Autodesk Inventor part; units mm, degrees
ref_plane "YZ Plane" through (0, 0, 0) normal (1, 0, 0) x (0, 1, 0)
ref_plane "XZ Plane" through (0, 0, 0) normal (0, 1, 0) x (-1, 0, 0)
ref_plane "XY Plane" through (0, 0, 0) normal (0, 0, 1) x (1, 0, 0)
sketch "Эскиз1" plane through (0, 0, 0) normal (0, 0, 1) x (1, 0, 0)
  line L0 (-25, 0) -> (25, 0) construction
  line L1 (-10, -2) -> (10, -2)
  line L2 (10, -2) -> (10, 2)
  line L3 (10, 2) -> (-10, 2)
  line L4 (-10, 2) -> (-10, -2)
  line L5 (-24, 5) -> (-20, 5)
  line L6 (-20, 5) -> (-20, -5)
  line L7 (-20, -5) -> (-24, -5)
  line L8 (-24, -5) -> (-24, 5)
  line L9 (0, 20) -> (0, -20) construction
  line L10 (24, 5) -> (20, 5)
  line L11 (20, 5) -> (20, -5)
  line L12 (20, -5) -> (24, -5)
  line L13 (24, -5) -> (24, 5)
  line L14 (-21, 20) -> (21, 20)
  line L15 (21, 20) -> (21, -20) construction
  line L16 (21, -20) -> (-21, -20)
  line L17 (-21, -20) -> (-21, 20) construction
  arc A0 (-21, 20) -> (-26, 15) centre (-21, 15) ccw
  arc A1 (-26, -15) -> (-21, -20) centre (-21, -15) ccw
  arc A2 (21, -20) -> (26, -15) centre (21, -15) ccw
  arc A3 (26, 15) -> (21, 20) centre (21, 15) ccw
  line L18 (-26, 15) -> (-26, -15)
  line L19 (26, -15) -> (26, 15)
  point P0 (0, 0)
  point P1 (-20, 0)
  point P2 (-10, 0)
  point P3 (0, -2)
  point P4 (0, 0)
  dimension "d0" = 4
  dimension "d1" = 40
  dimension "d2" = 20
  dimension "d3" = 10
  dimension "d4" = 50
  dimension "d6" = 52
  dimension "d7" = 40
  dimension "d8" = 5
extrude "Выдавливание1" add sketch "Эскиз1" along normal blind 4
properties part number "PistonPart5" material "Дерево (вишня)"
Here's how the part is built. I have some questions about the finished solid (model axes, mm). A direction names the side the tool comes from. Coordinates: 2 decimals unless noted, no trailing zeros. Write each loop counter-clockwise with the first axis right and the second up, starting at its lowest first coordinate (ties: lowest second). Pieces come first, ordered by that corner, then holes. Notation, with made-up numbers: (35.5, -19.5) -> (84.5, -19.5) arc R8 cw to (84.5, -4.5) -> close; hole circle Ø10 at (27.5, 77.5). An arc over 180 degrees is marked (long way). Use a Markdown table: item, result. Add a question column.
(1) I'm going to push a flat-ended pin straight in: P1, Ø2, axis at x = 21.5, z = 1.5, coming from the -Y side. Where does the tip first touch, or does it pass through?
(2) For faces 1 (the cylindrical face through (-25, 18, 2)), 2 (the flat face through (20, 0, 2)), which set-ups out of +Z, -Z, +X, -X, +Y, -Y let a thin tool reach every point of the face, with its end or its side?
(3) If we section it at C-C, the plane z = 1.5: Write out the boundary of the cut face in (x, y).
(4) If we section it at B-B, the plane y = 0: Write out the boundary of the cut face in (x, z).
(5) If we section it at A-A, the plane x = -7.5: Write out the boundary of the cut face in (y, z), and give its area (3 significant figures).
(6) Please list where these lines run through material, in increasing order: line 1 (X direction, y = 0.5, z = 3.75); line 2 (X direction, y = 2.5, z = 1.2); line 3 (Y direction, x = 7.5, z = 3.55).
(7) We'd pull the mould along Y, two halves only. Please class faces 3 (the flat face through (0, -2, 2)), 4 (the cylindrical face through (-24, -19, 2)), 5 (the flat face through (0, 20, 2)): +Y half, -Y half, draft (parallel to the pull), parting line (faces both ways), or undercut.
Outcome:
| question | item | result |
|---|---|---|
| 1 | P1 | stops at y = -20 |
| 2 | face 1 | +Z, -Z, -X, +Y |
| 2 | face 2 | +Z, -Z |
| 3 | outline | (-26, -15) arc R5 ccw to (-21, -20) -> (21, -20) arc R5 ccw to (26, -15) -> (26, 15) arc R5 ccw to (21, 20) -> (-21, 20) arc R5 ccw to (-26, 15) -> close; hole (-24, -5) -> (-20, -5) -> (-20, 5) -> (-24, 5) -> close; hole (-10, -2) -> (10, -2) -> (10, 2) -> (-10, 2) -> close; hole (20, -5) -> (24, -5) -> (24, 5) -> (20, 5) -> close |
| 4 | outline | (-26, 0) -> (-24, 0) -> (-24, 4) -> (-26, 4) -> close; (-20, 0) -> (-10, 0) -> (-10, 4) -> (-20, 4) -> close; (10, 0) -> (20, 0) -> (20, 4) -> (10, 4) -> close; (24, 0) -> (26, 0) -> (26, 4) -> (24, 4) -> close |
| 5 | outline | (-20, 0) -> (-2, 0) -> (-2, 4) -> (-20, 4) -> close; (2, 0) -> (20, 0) -> (20, 4) -> (2, 4) -> close |
| 5 | area | 144 mm^2 |
| 6 | line 1 | x = -26 to -24, -20 to -10, 10 to 20, 24 to 26 |
| 6 | line 2 | x = -26 to -24, -20 to 20, 24 to 26 |
| 6 | line 3 | y = -20 to -2, 2 to 20 |
| 7 | face 3 | undercut |
| 7 | face 4 | -Y half |
| 7 | face 5 | +Y half |
